Autodesk Inventor part; units mm, degrees
ref_plane "Work Plane1" through (-30.4574, 8.1557, 6.9453) normal (0, 0, -1) x (-1, 0, 0)
ref_plane "Work Plane2" through (0, 0, 6.9453) normal (0, 0, 1) x (1, 0, 0)
ref_plane "YZ Plane" through (0, 0, 0) normal (1, 0, 0) x (0, 1, 0)
sketch "Sketch1" plane through (0, 0, 0) normal (0, 0, 1) x (1, 0, 0)
  line L0 (-11.4074, 18.7393) -> (-11.4074, 6.0393)
  line L1 (-11.4074, 6.0393) -> (-30.4574, 6.0393)
  line L2 (-30.4574, 6.0393) -> (-30.4574, 10.8018)
  line L3 (-30.4574, 10.8018) -> (-24.1074, 18.7393)
  line L4 (-11.4074, 18.7393) -> (-24.1074, 18.7393)
  dimension "d0" = 12.7
  dimension "d1" = 19.05
  dimension "d2" = 4.7625
  dimension "d4" = 12.7
extrude "Extrusion1" add sketch "Sketch1" along normal blind 13.8906
sketch "Sketch3" plane through (-30.4574, 6.0393, 0) normal (-1, 0, 0) x (0, 0, 1)
  line L0 (13.8906, 0) -> (13.8906, 4.7625)
  line L1 (0, 4.7625) -> (13.8906, 4.7625)
  line L2 (0, 0) -> (0, 4.7625)
  line L3 (0, 0) -> (13.8906, 0)
  circle A0 centre (6.9453, 2.1164) radius 6.9453 construction
  line L4 (6.9453, 2.1164) -> (6.9453, 0)
ref_plane "Work Plane1" through (-30.4574, 8.1557, 6.9453) normal (0, 0, -1) x (-1, 0, 0)
sketch "Sketch4" plane through (-30.4574, 8.1557, 6.9453) normal (0, 0, -1) x (-1, 0, 0)
  line L0 (-4.7625, 8.2023) -> (0, 8.2023)
  line L1 (0, 8.2023) -> (0, 2.6461)
  line L2 (0, 2.6461) -> (-4.7625, 2.6461)
  line L3 (-4.7625, 2.6461) -> (-4.7625, 8.2023)
  line L4 (0, -2.1164) -> (0, 2.6461)
  dimension "d13" = 4.7625
  dimension "d14" = 5.5563
extrude "Extrusion3" cut sketch "Sketch4" against normal mid plane 9.525
sketch "Sketch5" plane through (-11.4074, 6.0393, 0) normal (1, 0, 0) x (0, 0, -1)
  line L0 (-13.8906, 12.7) -> (-13.8906, 0)
  line L1 (0, 0) -> (-13.8906, 0)
  line L2 (0, 12.7) -> (0, 0)
  line L3 (0, 12.7) -> (-13.8906, 12.7)
  line L4 (-11.7078, 9.525) -> (-2.1828, 9.525)
  line L5 (-2.1828, 9.525) -> (-2.1828, 3.175)
  line L6 (-2.1828, 3.175) -> (-11.7078, 3.175)
  line L7 (-11.7078, 3.175) -> (-11.7078, 9.525)
  circle A0 centre (-6.9453, 6.35) radius 4.7625 construction
  circle A1 centre (-6.9453, 6.35) radius 3.175 construction
  circle A2 centre (-6.9453, 6.35) radius 6.35 construction
  circle A3 centre (-6.9453, 6.35) radius 6.9453 construction
  dimension "d17" = 9.525
  dimension "d18" = 6.35
extrude "Extrusion4" cut sketch "Sketch5" against normal blind 12.7 contours L4 L5 L6 L7
sketch "Sketch6" plane through (-11.4074, 6.0393, 0) normal (1, 0, 0) x (0, 0, -1)
  line L0 (-11.7078, 3.175) -> (-11.7078, 9.525)
  line L1 (-11.7078, 9.525) -> (-2.1828, 9.525)
  line L2 (-2.1828, 9.525) -> (-2.1828, 3.175)
  line L3 (-10.1203, 9.525) -> (-3.7703, 9.525)
  line L4 (-3.7703, 9.525) -> (-3.7703, 11.1125)
  line L5 (-3.7703, 11.1125) -> (-10.1203, 11.1125)
  line L6 (-10.1203, 11.1125) -> (-10.1203, 9.525)
  circle A0 centre (-6.9453, 20.5431) radius 3.175 construction
  circle A1 centre (-6.9453, 20.5431) radius 4.7625 construction
  dimension "d21" = 6.35
  dimension "d22" = 1.5875
extrude "Extrusion5" cut sketch "Sketch6" against normal blind 3.175
sketch "Sketch7" plane through (-11.4074, 6.0393, 0) normal (1, 0, 0) x (0, 0, -1)
  line L0 (-13.8906, 12.7) -> (-13.8906, 0)
  line L1 (0, 0) -> (-13.8906, 0)
  line L2 (0, 12.7) -> (0, 0)
  line L3 (0, 12.7) -> (-13.8906, 12.7)
  line L4 (-12.5016, 7.9375) -> (-1.3891, 7.9375)
  line L5 (-1.3891, 7.9375) -> (-1.3891, 4.7625)
  line L6 (-1.3891, 4.7625) -> (-12.5016, 4.7625)
  line L7 (-12.5016, 4.7625) -> (-12.5016, 7.9375)
  circle A0 centre (-6.9453, 6.35) radius 5.5563 construction
  circle A1 centre (-6.9453, 6.35) radius 6.9453 construction
  circle A2 centre (-6.9453, 6.35) radius 6.35 construction
  circle A3 centre (-6.9453, 6.35) radius 1.5875 construction
  dimension "d25" = 3.175
  dimension "d26" = 11.1125
extrude "Extrusion6" cut sketch "Sketch7" against normal blind 9.525 contours L4 L5 L6 L7
sketch "Sketch8" plane through (-11.4074, 6.0393, 0) normal (1, 0, 0) x (0, 0, -1)
  line L0 (-10.1203, 9.525) -> (-10.1203, 11.1125)
  line L1 (-3.7703, 11.1125) -> (-3.7703, 9.525)
  line L2 (-2.1828, 3.175) -> (-11.7078, 3.175)
  line L3 (-10.1203, 3.175) -> (-3.7703, 3.175)
  line L4 (-3.7703, 3.175) -> (-3.7703, 1.5875)
  line L5 (-3.7703, 1.5875) -> (-10.1203, 1.5875)
  line L6 (-10.1203, 1.5875) -> (-10.1203, 3.175)
  dimension "d29" = 1.5875
extrude "Extrusion7" cut sketch "Sketch8" against normal up to surface (12.7 mm away)
sketch "Sketch9" plane through (-30.4574, 6.0393, 0) normal (0, -1, 0) x (1, 0, 0)
  line L0 (19.05, 13.8906) -> (0, 13.8906)
  line L1 (19.05, 0) -> (0, 0)
  line L2 (19.05, 0) -> (19.05, 13.8906)
  line L3 (11.5094, -0.1544) -> (11.5094, 2.9198)
  line L4 (11.5094, 10.9708) -> (11.5094, 14.045)
  line L5 (10.7156, -0.1544) -> (10.7156, 2.9198)
  line L6 (10.7156, 10.9708) -> (10.7156, 14.045)
  arc A0 (10.7156, 2.9198) -> (10.7156, -0.1544) centre (11.1125, 1.3827) ccw
  arc A1 (11.5094, -0.1544) -> (11.5094, 2.9198) centre (11.1125, 1.3827) ccw
  arc A2 (11.5094, 10.9708) -> (11.5094, 14.045) centre (11.1125, 12.5079) ccw
  arc A3 (10.7156, 14.045) -> (10.7156, 10.9708) centre (11.1125, 12.5079) ccw
  circle A4 centre (11.1125, 6.9453) radius 5.5626 construction
  circle A5 centre (11.1125, 6.9453) radius 6.9453 construction
  dimension "d32" = 7.9375
  dimension "d33" = 1.5875
  dimension "d34" = 0.7937
  dimension "d35" = 0.3969
  dimension "d45" = 11.1252
extrude "Extrusion8" add sketch "Sketch9" along normal blind 3.175
sketch "Sketch10" plane through (-24.1074, 18.7393, 0) normal (0, 1, 0) x (1, 0, 0)
  line L0 (0, -13.8906) -> (12.7, -13.8906)
  line L1 (12.7, 0) -> (12.7, -13.8906)
  line L2 (0, 0) -> (12.7, 0)
  line L3 (9.525, 0) -> (-3.175, 0)
  line L4 (-3.175, 0) -> (-3.175, -2.3813)
  line L5 (-3.175, -2.3813) -> (9.525, -2.3812)
  line L6 (9.525, -2.3812) -> (9.525, 0)
  line L7 (9.525, -11.5094) -> (-3.175, -11.5094)
  line L8 (-3.175, -11.5094) -> (-3.175, -13.8906)
  line L9 (-3.175, -13.8906) -> (9.525, -13.8906)
  line L10 (9.525, -13.8906) -> (9.525, -11.5094)
  dimension "d38" = 3.175
  dimension "d39" = 2.3813
  dimension "d40" = 2.3813
  dimension "d41" = 12.7
  dimension "d42" = 12.7
extrude "Extrusion9" cut sketch "Sketch10" against normal blind 1.27
ref_plane "Work Plane2" through (0, 0, 6.9453) normal (0, 0, 1) x (1, 0, 0)
sketch "Sketch12" plane through (0, 0, 6.9453) normal (0, 0, 1) x (1, 0, 0)
  line L0 (-34.925, 19.05) -> (-7.9375, 19.05)
  line L1 (-7.9375, 19.05) -> (-7.9375, -1.5875)
  line L2 (-7.9375, -1.5875) -> (-34.925, -1.5875)
  line L3 (-34.925, -1.5875) -> (-34.925, 19.05)
extrude "Extrusion10" cut sketch "Sketch12" along normal through all
properties part number "connect"
For this review, take the finished solid that the model builds, in its own axes (mm). A direction names the side the tool comes from. Round coordinates to 2 decimals unless told otherwise and drop trailing zeros. Loops run counter-clockwise (first coordinate to the right, second up) from the corner with the lowest first, then second, coordinate; pieces in that order, holes last.
(1) We need section A-A (z = 3.5). Give the boundary of the cut face in (x, y).
Returned:
outline: (-30.46, 6.04) - (-11.41, 6.04) - (-11.41, 9.21) - (-24.11, 9.21) - (-24.11, 15.56) - (-11.41, 15.56) - (-11.41, 18.74) - (-24.11, 18.74) - (-26.01, 16.36) - (-25.69, 16.36) - (-25.69, 10.8) - (-30.46, 10.8) - close
(2) We need section C-C (y = 9.75). Give the boundary of the cut face in (x, z), plus the area to 3 significant figures.
Returned:
outline: (-30.46, 0) - (-11.41, 0) - (-11.41, 2.18) - (-24.11, 2.18) - (-24.11, 6.95) - (-30.46, 6.95) - close
area: 71.8 mm2
(3) We need section B-B (x = -13.5). Give the boundary of the cut face in (y, z), plus the area to 3 significant figures.
Returned:
outline: (6.04, 0) - (18.74, 0) - (18.74, 6.95) - (17.15, 6.95) - (17.15, 3.77) - (15.56, 3.77) - (15.56, 2.18) - (13.98, 2.18) - (13.98, 1.39) - (10.8, 1.39) - (10.8, 2.18) - (9.21, 2.18) - (9.21, 3.77) - (7.63, 3.77) - (7.63, 6.95) - (6.04, 6.95) - close
area: 45.4 mm2
(4) Tool access review of faces 1 (the flat face through (-20, 17.469, 1)), 2 (the flat face through (-26.62, 15.6, 1.88)), 3 (the flat face through (-13, 17.152, 5)), 4 (the flat face through (-25.695, 14, 5)), 5 (the flat face through (-25, 12, 6.945)): name each direction out of +Z, -Z, +X, -X, +Y, -Y from which nothing blocks a thin tool from reaching the whole face with its end or side.
Returned:
face 1: -Z, -X, +Y
face 2: +Z, -Z, -X, +Y
face 3: +Z, +X
face 4: +Z, -X
face 5: +Z, +X, -X, +Y, -Y
(5) Clearance check with flat-ended pins moving along their axes: P1, Ø1.6, axis at x = -17.5, y = 11.5, coming from the +Z side; P2, Ø1.4, axis at y = 18, z = 1.5, coming from the -X side; P3, Ø2.5, axis at x = -17.5, z = 0.5, coming from the +Y side. State where each tip first meets the part, or that it passes through.
Returned:
P1: stops at z = 2.18
P2: stops at x = -25.26
P3: stops at y = 17.47
(6) Mouldability with a two-part tool opening along X and no side actions: class faces 6 (the flat face through (-18, 9.214, 3)), 7 (the flat face through (-18.948, 4, 1)), 8 (the flat face through (-14.582, 18, 1)), 9 (the flat face through (-19.742, 4, 1)) as released by +X, released by -X, zero draft, split by the parting line, or undercut.
Returned:
face 6: zero draft
face 7: undercut
face 8: released by -X
face 9: undercut
(7) Wall thickness on line 1 along Y through (x, z) = (-23.25, 2.5); line 2 along Y through (x, z) = (-20.75, 4.5); line 3 along X through (y, z) = (7.75, 5.25): over which ranges is each line inside the solid? List them lowest first.
Returned:
line 1: y = 6.04 to 9.21, 15.56 to 18.74
line 2: y = 6.04 to 7.63, 15.56 to 18.74
line 3: x = -30.46 to -24.11
(8) We need section D-D (z = 6.5). Give the boundary of the cut face in (x, y), plus the area to 3 significant figures.
Returned:
outline: (-30.46, 6.04) - (-11.41, 6.04) - (-11.41, 7.63) - (-24.11, 7.63) - (-24.11, 15.56) - (-14.58, 15.56) - (-14.58, 17.15) - (-11.41, 17.15) - (-11.41, 18.74) - (-24.11, 18.74) - (-26.01, 16.36) - (-25.69, 16.36) - (-25.69, 10.8) - (-30.46, 10.8) - close
area: 96.8 mm2
